Autodesk Inventor part; units mm, degrees
ref_plane "YZ Plane" through (0, 0, 0) normal (1, 0, 0) x (0, 1, 0)
ref_plane "XZ Plane" through (0, 0, 0) normal (0, 1, 0) x (-1, 0, 0)
ref_plane "XY Plane" through (0, 0, 0) normal (0, 0, 1) x (1, 0, 0)
sketch "Sketch1" plane through (0, 0, 0) normal (0, 0, 1) x (1, 0, 0)
  circle A0 centre (0, 0) radius 20.32
  dimension "d0" = 40.64
extrude "Extrusion1" add sketch "Sketch1" along normal blind 45.72
sketch "Sketch2" plane through (0, 0, 0) normal (0, 0, -1) x (-1, 0, 0)
  circle A0 centre (0, 0) radius 19.05
  circle A1 centre (0, 0) radius 20.32
  dimension "d3" = 38.1
extrude "Extrusion2" cut sketch "Sketch2" against normal blind 40.64 contours A0
sketch "Sketch3" plane through (0, 0, 40.64) normal (0, 0, -1) x (-1, 0, 0)
  arc A0 (16.51, 2.54) -> (16.51, -2.54) centre (16.51, 0) ccw
  circle A1 centre (0, 0) radius 19.05
  line L0 (16.51, 2.54) -> (18.8799, 2.54)
  line L1 (16.51, -2.54) -> (18.8799, -2.54)
  arc A2 (18.8799, -2.54) -> (18.8799, 2.54) centre (0, 0) ccw
  line L2 (2.6862, 16.4868) -> (3.4185, 18.7408)
  arc A3 (8.2499, 17.171) -> (3.4185, 18.7408) centre (0, 0) ccw
  line L3 (7.5176, 14.917) -> (8.2499, 17.171)
  arc A4 (2.6862, 16.4868) -> (7.5176, 14.917) centre (5.1019, 15.7019) ccw
  line L4 (-14.8498, 7.6494) -> (-16.7671, 9.0424)
  arc A5 (-13.7812, 13.1522) -> (-16.7671, 9.0424) centre (0, 0) ccw
  line L5 (-11.8639, 11.7592) -> (-13.7812, 13.1522)
  arc A6 (-14.8498, 7.6494) -> (-11.8639, 11.7592) centre (-13.3569, 9.7043) ccw
  line L6 (-11.8639, -11.7592) -> (-13.7812, -13.1522)
  arc A7 (-16.7671, -9.0424) -> (-13.7812, -13.1522) centre (0, 0) ccw
  line L7 (-14.8498, -7.6494) -> (-16.7671, -9.0424)
  arc A8 (-11.8639, -11.7592) -> (-14.8498, -7.6494) centre (-13.3569, -9.7043) ccw
  line L8 (7.5176, -14.917) -> (8.2499, -17.171)
  arc A9 (3.4185, -18.7408) -> (8.2499, -17.171) centre (0, 0) ccw
  line L9 (2.6862, -16.4868) -> (3.4185, -18.7408)
  arc A10 (7.5176, -14.917) -> (2.6862, -16.4868) centre (5.1019, -15.7019) ccw
  dimension "d6" = 5.08
  dimension "d9" = 360
extrude "Extrusion3" add sketch "Sketch3" along normal up to surface (40.64 mm away) contours L0 A1 L1 A0 | L3 A4 L2 A1 | A1 L9 A10 L8 | L5 A6 L4 A1 | A1 L7 A8 L6
sketch "Sketch4" plane through (0, 0, 0) normal (0, 0, -1) x (-1, 0, 0)
  arc A0 (16.51, 2.54) -> (16.51, -2.54) centre (16.51, 0) ccw
  circle A1 centre (16.51, 0) radius 1.524
  circle A2 centre (5.1019, 15.7019) radius 1.524
  circle A3 centre (-13.3569, 9.7043) radius 1.524
  circle A4 centre (-13.3569, -9.7043) radius 1.524
  circle A5 centre (5.1019, -15.7019) radius 1.524
  point P0 (0, 0)
  dimension "d13" = 3.048
  dimension "d16" = 360
extrude "Extrusion4" cut sketch "Sketch4" against normal blind 33.02
fillet "Fillet1" radius 7.62 1 edges at (-20.32, 0, 45.72)
fillet "Fillet2" radius 3.175 1 edges at (-18.8799, -2.54, 20.32)
properties part number "MetalFrame"
Geometry check sheet. Reference: the model listing, model coordinates, mm. Round coordinates to 2 decimals unless told otherwise and drop trailing zeros. Loops run counter-clockwise (first coordinate to the right, second up) from the corner with the lowest first, then second, coordinate; pieces in that order, holes last. Notation, with made-up numbers: (61.5, -39) - (111.5, -39) arc R15 ccw to (111.5, -29) - close; hole circle Ø4 at (1, 29). An arc over 180 degrees is marked (long way). Use a Markdown table: item, result.
Q1. Cross-section at B-B on x = 0. Record the cut outline in (y, z).
Solutions:
| item | result |
|---|---|
| outline | (-20.32, 0) - (-19.05, 0) - (-19.05, 40.64) - (19.05, 40.64) - (19.05, 0) - (20.32, 0) - (20.32, 38.1) arc R7.62 ccw to (12.7, 45.72) - (-12.7, 45.72) arc R7.62 ccw to (-20.32, 38.1) - close |
Q2. Cross-section at A-A on y = 0. Record the cut outline in (x, z).
Solutions:
| item | result |
|---|---|
| outline | (-20.32, 0) - (-18.03, 0) - (-18.03, 33.02) - (-14.99, 33.02) - (-14.99, 0) - (-13.97, 0) - (-13.97, 40.64) - (19.05, 40.64) - (19.05, 0) - (20.32, 0) - (20.32, 38.1) arc R7.62 ccw to (12.7, 45.72) - (-12.7, 45.72) arc R7.62 ccw to (-20.32, 38.1) - close |
Q3. Cross-section at D-D on z = 42.5. Record the cut outline in (x, y), plus the area to 3 significant figures.
Solutions:
| item | result |
|---|---|
| outline | circle Ø37.84 at (0, 0) |
| area | 1,120 mm2 |
Q4. Material ranges on line 1 (Y direction, x = -14.5, z = 37); line 2 (X direction, y = 15, z = 16); line 3 (X direction, y = -16, z = 18), recorded low to high.
Solutions:
| item | result |
|---|---|
| line 1 | y = -14.24 to -12.36, -1.55 to 1.55, 12.36 to 14.24 |
| line 2 | x = -13.71 to -11.74, -7.54 to -6.45, -3.75 to -2.66, 11.74 to 13.71 |
| line 3 | x = -12.53 to -10.34, -7.87 to -6.6, -3.61 to -2.58, 10.34 to 12.53 |
Q5. Cross-section at C-C on z = 25. State how many separate pieces and enclosed holes the cut face has, plus the area to 3 significant figures.
Solutions:
| item | result |
|---|---|
| separate pieces | 1 |
| enclosed holes | 6 |
| area | 238 mm2 |
Q6. Go/stop test with flat-tipped pins: P1, Ø10, axis at y = -10, z = 38.5, coming from the -X side; P2, Ø5, axis at y = -8, z = 31.5, coming from the -X side; P3, Ø4, axis at x = 13.36, y = 9.7, coming from the +Z side. Record where each tip stops, or that it passes through.
Solutions:
| item | result |
|---|---|
| P1 | stops at x = -19.69 |
| P2 | stops at x = -19.56 |
| P3 | stops at z = 45.5 |
